Source: CAD feature listing. Evaluate the final solid. Frame: model axes, mm. A direction names the side the tool comes from. Give positions to 0.01 mm unless a question says otherwise; leave off trailing zeros. Loops run counter-clockwise (first coordinate to the right, second up) from the corner with the lowest first, then second, coordinate; pieces in that order, holes last. Notation, with made-up numbers: M -31.5,-27.75 L 17.5,-27.75 A27 cw 17.5,-2.75 Z; hole C 77.5,-4.75 d8. An arc over 180 degrees is marked long. Answer in a Markdown table with one row per item.
```python
from build123d import *

# Parameters (mm, degrees)
SKETCH_1_W           = 22.72
SKETCH_1_H           = 9
EXTRUDE_1_DEPTH      = 9
SKETCH_2_W           = 20.32
SKETCH_2_H           = 6.6
CUT_EXTRUDE_1_DEPTH  = 6.5
SKETCH_3_W           = 4.2
SKETCH_3_H           = 6.5
CUT_EXTRUDE_2_DEPTH  = 6.5
EXTRUDE_2_DEPTH      = 3.5
EXTRUDE_2_DEPTH_BACK = 8
SKETCH_5_W           = 0.75
SKETCH_5_H           = 0.75


with BuildPart() as part:
    # 草图1 → 拉伸1 (new body)
    with BuildSketch(Plane(origin=(0, 0, 0), x_dir=(1, 0, 0), z_dir=(0, 1, 0))):
        Rectangle(SKETCH_1_W, SKETCH_1_H)
    extrude(amount=EXTRUDE_1_DEPTH)

    # 草图2 → 切除-拉伸1 (cut)
    with BuildSketch(Plane(origin=(0, 9, 0), x_dir=(-1, 0, 0), z_dir=(0, 1, 0))):
        Rectangle(SKETCH_2_W, SKETCH_2_H)
    extrude(amount=-CUT_EXTRUDE_1_DEPTH, mode=Mode.SUBTRACT)

    # 草图3 → 切除-拉伸2 (cut)
    with BuildSketch(Plane.XY.offset(4.5)):
        with Locations((0, 5.75)):
            Rectangle(SKETCH_3_W, SKETCH_3_H)
    extrude(amount=-CUT_EXTRUDE_2_DEPTH, mode=Mode.SUBTRACT)

    # 草图5 → 拉伸2 (add, two sides: drawn at the far end of the back side and taken through both)
    with BuildSketch(Plane.XZ.offset(-EXTRUDE_2_DEPTH_BACK)):
        with Locations((-1.27, 1.27)):
            Rectangle(SKETCH_5_W, SKETCH_5_H)
        with Locations((-3.81, 1.27)):
            Rectangle(SKETCH_5_W, SKETCH_5_H)
        with Locations((-6.35, 1.27)):
            Rectangle(SKETCH_5_W, SKETCH_5_H)
        with Locations((-6.35, -1.27)):
            Rectangle(SKETCH_5_W, SKETCH_5_H)
        with Locations((-3.81, -1.27)):
            Rectangle(SKETCH_5_W, SKETCH_5_H)
        with Locations((-1.27, -1.27)):
            Rectangle(SKETCH_5_W, SKETCH_5_H)
        with Locations((1.27, -1.27)):
            Rectangle(SKETCH_5_W, SKETCH_5_H)
        with Locations((3.81, -1.27)):
            Rectangle(SKETCH_5_W, SKETCH_5_H)
        with Locations((6.35, -1.27)):
            Rectangle(SKETCH_5_W, SKETCH_5_H)
        with Locations((6.35, 1.27)):
            Rectangle(SKETCH_5_W, SKETCH_5_H)
        with Locations((3.81, 1.27)):
            Rectangle(SKETCH_5_W, SKETCH_5_H)
        with Locations((1.27, 1.27)):
            Rectangle(SKETCH_5_W, SKETCH_5_H)
    extrude(amount=EXTRUDE_2_DEPTH + EXTRUDE_2_DEPTH_BACK)


solid = part.part
```
1) Pull-direction query (X, two-part tool) for faces 1 (the flat face through (11.36, 4, 0)), 2 (the flat face through (-10.16, 6, 0)), 3 (the flat face through (0, 2, 4.5)), 4 (the flat face through (-11.36, 4, 0)); classes: released by +X, released by -X, zero draft, split by the parting line, or undercut.
Reply:
| item | result |
|---|---|
| face 1 | released by +X |
| face 2 | undercut |
| face 3 | zero draft |
| face 4 | released by -X |
2) Material intervals for L1, parallel to Z at x = -3.75, y = 7 (3 decimals); L2, parallel to X at y = 4.5, z = -1.75; L3, parallel to X at y = 8, z = 3.5, sorted ascending.
Reply:
| item | result |
|---|---|
| L1 | z = -4.5 to -3.3, -1.645 to -0.895, 0.895 to 1.645, 3.3 to 4.5 |
| L2 | x = -11.36 to -10.16, 10.16 to 11.36 |
| L3 | x = -11.36 to -2.1, 2.1 to 11.36 |
3) Section C-C, the plane y = 5. Count the separate pieces of the cut face and the enclosed holes in it, then the cut area to 3 significant figures.
Reply:
| item | result |
|---|---|
| separate pieces | 13 |
| enclosed holes | 0 |
| area | 72.1 mm² |
4) Section B-B, the plane z = 4. Return loops of the section in (x, y), then the cut area to 3 significant figures.
Reply:
| item | result |
|---|---|
| outline | M -11.36,0 L 11.36,0 L 11.36,9 L 2.1,9 L 2.1,2.5 L -2.1,2.5 L -2.1,9 L -11.36,9 Z |
| area | 177 mm² |
5) Set-up query: faces 5 (the flat face through (-1, 9, -4)), 6 (the flat face through (-6, 6, 3.3)), 7 (the flat face through (-2.1, 6, 4)). Return all of +Z, -Z, +X, -X, +Y, -Y with unobstructed straight access to the full face (end or side cutting, diameter ignored); none if empty.
Reply:
| item | result |
|---|---|
| face 5 | +Z, -Z, +X, -X, +Y |
| face 6 | +Y |
| face 7 | +Z, +Y |
6) Section A-A, the plane x = 5.25. Return loops of the section in (y, z).
Reply:
| item | result |
|---|---|
| outline | M 0,-4.5 L 9,-4.5 L 9,-3.3 L 2.5,-3.3 L 2.5,3.3 L 9,3.3 L 9,4.5 L 0,4.5 Z |
7) Pin query (flat end, axial travel): pin 1 Ø0.6 at (x, y) = (-6.5, -2) entering from +Z (3 decimals); pin 2 Ø0.8 at (x, y) = (6.5, -1.5) entering from -Z (3 decimals); pin 3 Ø1 at (y, z) = (-2, -1) entering from -X (3 decimals). Return the tip coordinate at first contact, or that it passes through.
Reply:
| item | result |
|---|---|
| pin 1 | stops at z = 1.645 |
| pin 2 | stops at z = -1.645 |
| pin 3 | stops at x = -6.725 |
